```python
from build123d import *

# Parameters (mm, degrees)
SKETCH1_W           = 15.875
SKETCH1_H           = 22.225
BOSS_EXTRUDE1_DEPTH = 4.7625
SKETCH2_W           = 6.35
SKETCH2_H           = 22.225
CUT_EXTRUDE1_DEPTH  = 3.175
SKETCH3_R           = 31.75
CUT_EXTRUDE2_DEPTH  = 50.924287989
CHAMFER1_SIZE       = 2.23064129
CHAMFER1_SIZE_2     = 2.54
SKETCH4_R           = 1.55
CUT_EXTRUDE3_DEPTH  = 47.797604439
FILLET1_R           = 1.5875


with BuildPart() as part:
    # Sketch1 → Boss-Extrude1 (new, symmetric)
    with BuildSketch(Plane.XY):
        with Locations((-36.5125, 0)):
            Rectangle(SKETCH1_W, SKETCH1_H)
    extrude(amount=BOSS_EXTRUDE1_DEPTH, both=True)

    # Sketch2 → Cut-Extrude1 (cut, symmetric)
    with BuildSketch(Plane.XY):
        with Locations((-41.275, 0)):
            Rectangle(SKETCH2_W, SKETCH2_H)
    extrude(amount=CUT_EXTRUDE1_DEPTH, both=True, mode=Mode.SUBTRACT)

    # Sketch3 → Cut-Extrude2 (cut, through all)
    with BuildSketch(Plane(origin=(0, 11.1125, 0), x_dir=(1, 0, 0), z_dir=(0, 1, 0))):
        Circle(SKETCH3_R)
    extrude(amount=-CUT_EXTRUDE2_DEPTH, mode=Mode.SUBTRACT)

    # Chamfer1
    # the kernel refuses this chamfer: 2.54, 2.23064129 mm, written as the material it takes off along each edge
    with BuildSketch(Plane(origin=(-31.390780394, -17.93455078, -4.7625), x_dir=(-1, 0, 0), z_dir=(0, 1, 0))) as chamfer1_piece_1:
        with BuildLine():
            Line((CHAMFER1_SIZE, 0), (0.288027051, 2.637492029))
            ThreePointArc((0.288027051, 2.637492029), (0.17562072, 1.352980867), (0, 0))
            Line((0, 0), (CHAMFER1_SIZE, 0))
        make_face()
    extrude(amount=35.86910156, mode=Mode.SUBTRACT)
    with BuildSketch(Plane(origin=(-31.390780394, -17.644574789, 4.7625), x_dir=(-1, 0, 0), z_dir=(0, 1, 0))) as chamfer1_piece_2:
        with BuildLine():
            Line((CHAMFER1_SIZE_2, 0), (0.261871886, -2.278128114))
            ThreePointArc((0.261871886, -2.278128114), (0.155107804, -1.168138054), (0, 0))
            Line((0, 0), (CHAMFER1_SIZE_2, 0))
        make_face()
    extrude(amount=35.289149579, mode=Mode.SUBTRACT)
    with BuildSketch(Plane(origin=(0, 11.1125, 0), x_dir=(-0.9371917542835735, 0, -0.34881458642504903), z_dir=(0.34881458642504903, 0, -0.9371917542835735))) as chamfer1_piece_3:
        Polygon((31.75 + CHAMFER1_SIZE_2, 0), (31.75, -CHAMFER1_SIZE_2), (31.75, 0), align=None)
    revolve(axis=Axis((0, 11.1125, 0), (0, 1, 0)), revolution_arc=40.829654119, mode=Mode.SUBTRACT)

    # Sketch4 → Cut-Extrude3 (cut, through all)
    with BuildSketch(Plane.XY.offset(4.7625)):
        with Locations((-41.275, 0)):
            Circle(SKETCH4_R)
    extrude(amount=-CUT_EXTRUDE3_DEPTH, mode=Mode.SUBTRACT)

    # Fillet1
    fillet1_edges = [part.edges().sort_by_distance(p)[0] for p in [
        (-44.45, -11.1125, -3.96875),
        (-44.45, 11.1125, -3.96875),
        (-44.45, -11.1125, 3.96875),
        (-44.45, 11.1125, 3.96875),
    ]]
    fillet(fillet1_edges, radius=FILLET1_R)


solid = part.part
```
Could you check a few things on this model? Use its own coordinates, in mm. A direction names the side the tool comes from. Round coordinates to 2 decimals unless told otherwise and drop trailing zeros. Order: outer loops, then holes, each group sorted by start corner. A loop starts at its lowest first (then second) coordinate and runs counter-clockwise, first axis right, second up. Notation, with made-up numbers: M 29.5,-31.75 L 47.5,-31.75 A23 ccw 47.5,2.25 Z; hole C 29,75.25 d7. An arc over 180 degrees is marked long. One line per question, with ' | ' between items. Start each with the question number.
(1) Suppose I cut it at B-B on x = -39. List the corners of the cut face in (y, z) for me (1 decimal), then the cut area to 3 significant figures.
(2) Suppose I cut it at C-C on z = 0. List the corners of the cut face in (x, y) for me, then the cut area to 3 significant figures.
(3) For faces 5 (the face through (-43.997, 10.635, -3.98)), 6 (the face through (-39, 0, -3.175)), which set-ups out of +Z, -Z, +X, -X, +Y, -Y let a thin tool reach every point of the face, with its end or its side?
(4) Suppose I cut it at A-A on y = 0. Count the separate pieces of the cut face and the enclosed holes in it, then the cut area to 3 significant figures.
(5) Please list where these lines run through material, in increasing order: line 1 along Z through (x, y) = (-41.75, -9) (1 decimal); line 2 along X through (y, z) = (7, 0.25); line 3 along Y through (x, z) = (-40.75, 3.75).
(6) For P1, Ø3, axis at y = 0, z = -3, coming from the +X side, with a flat end and sliding along its axis, tell me the tip position at first contact or that it passes through.
(7) Thinking about a two-plate mould opening in Y: for faces 1 (the face through (-36, -11.112, 0)), 2 (the face through (-39.8, 0.47, -3.96)), 3 (the face through (-39.8, 0.47, 3.98)), 4 (the face through (-32.81, -0.17, 3.64)), which applies, +Y half, -Y half, draft (parallel to the pull), parting line (faces both ways), or undercut?
Geometry results:
1) outline: M -11.1,-4.8 L 11.1,-4.8 L 11.1,-3.2 L -11.1,-3.2 Z; M -11.1,3.2 L 11.1,3.2 L 11.1,4.8 L -11.1,4.8 Z | area: 70.6 mm²
2) outline: M -38.1,-11.11 L -31.75,-11.11 L -31.75,8.57 L -34.29,11.11 L -38.1,11.11 Z | area: 138 mm²
3) face 5: +Z, -Z, -X, +Y | face 6: -X, +Y, -Y
4) separate pieces: 3 | enclosed holes: 0 | area: 66.2 mm²
5) line 1: -4.8 to -3.2, 3.2 to 4.8 | line 2: -38.1 to -31.75 | line 3: -11.11 to -1.46, 1.46 to 11.11
6) P1: x = -31.68
7) face 1: -Y half | face 2: undercut | face 3: undercut | face 4: draft
